Geometry: see drawing. Coordinates: mm, zero at the bounding-box minimum. A direction names the side the tool comes from. Round coordinates to 2 decimals unless told otherwise and drop trailing zeros. Loops run counter-clockwise (first coordinate to the right, second up) from the corner with the lowest first, then second, coordinate; pieces in that order, holes last. Notation, with made-up numbers: (31.25, 75.5) - (36.25, 75.5) arc R19 cw to (36.25, 96.5) - close; hole circle Ø2 at (65, 34). An arc over 180 degrees is marked (long way). Write item = value, one per line. Start each with the question number.
Item 1: Draft query along X for the marked faces 1, 2, 3 and 4. Return one class per face: pulls with the +X half, pulls with the -X half, needs draft (parallel to the pull), parting line crosses it, or undercut.
Item 2: Access query for the marked faces 5 and 6. Directions: +Z, -Z, +X, -X, +Y, -Y. A direction counts if a zero-diameter tool reaches every point of the face in a straight line with its end or side. Return the directions, or none.
Item 3: Line query: line 1 (X direction, y = 56, z = 5.5); line 2 (Y direction, x = 4.5, z = 33); line 3 (Y direction, x = 50, z = 22). Output: solid intervals per line, ascending. Write a range as from..to.
Item 4: First-contact query: pin 1 (2.5 mm diameter, centred on x = 11, z = 16.5, fed in from +Y); pin 2 (2 mm diameter, centred on x = 43.5, z = 35, fed in from -Y); pin 3 (2 mm diameter, centred on y = 14, z = 31.5, fed in from -X); pin 4 (10.5 mm diameter, centred on y = 41.5, z = 14.5, fed in from +X). Flat tips, straight axial feed; report the tip coordinate or a pass-through.
Item 5: Section C-C (x = 28). Return loops of the section in (y, z).
Item 6: Section A-A (z = 16.5). Count the separate pieces of the cut face and the enclosed holes in it, plus the area to 3 significant figures.
Item 7: Section D-D (y = 67). Return loops of the section in (x, z).
Item 8: Section B-B (y = 49). Return loops of the section in (x, z), plus the area to 3 significant figures.
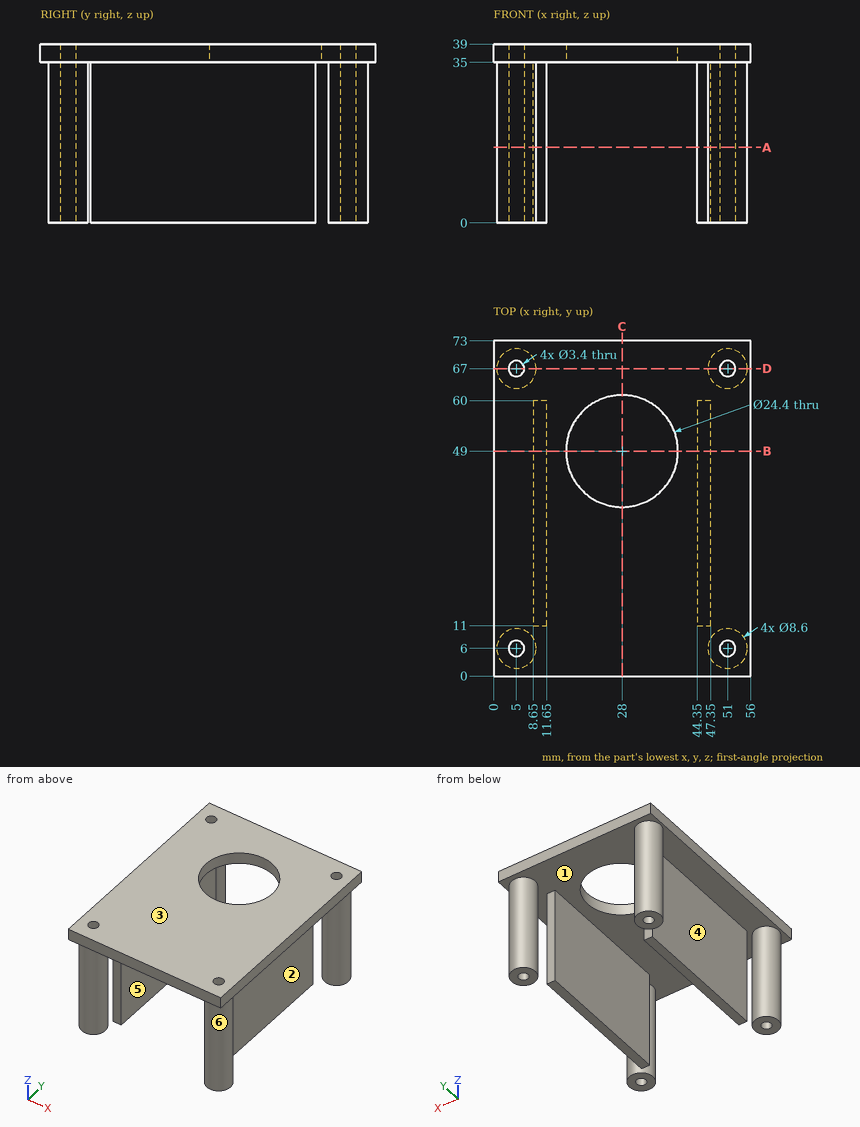
Taken from the geometry:
q1.face_1 = undercut
q1.face_2 = pulls with the +X half
q1.face_3 = needs draft
q1.face_4 = pulls with the -X half
q2.face_5 = -Z, +Y, -Y
q2.face_6 = -Z
q3.line_1 = 8.65..11.65, 44.35..47.35
q3.line_2 = 1.73..4.38, 7.62..10.27, 62.73..65.38, 68.62..71.27
q3.line_3 = 1.82..4.63, 7.37..10.18, 62.82..65.63, 68.37..71.18
q4.pin_1 = 60
q4.pin_2 = 0
q4.pin_3 = 8.65
q4.pin_4 = 47.35
q5.outline = (0, 35) - (36.8, 35) - (36.8, 39) - (0, 39) - close; (61.2, 35) - (73, 35) - (73, 39) - (61.2, 39) - close
q6.separate_pieces = 6
q6.enclosed_holes = 4
q6.area = 490 mm^2
q7.outline = (0, 35) - (0.7, 35) - (0.7, 0) - (3.3, 0) - (3.3, 39) - (0, 39) - close; (6.7, 0) - (9.3, 0) - (9.3, 35) - (46.7, 35) - (46.7, 0) - (49.3, 0) - (49.3, 39) - (6.7, 39) - close; (52.7, 0) - (55.3, 0) - (55.3, 35) - (56, 35) - (56, 39) - (52.7, 39) - close
q8.outline = (0, 35) - (8.65, 35) - (8.65, 0) - (11.65, 0) - (11.65, 35) - (15.8, 35) - (15.8, 39) - (0, 39) - close; (40.2, 35) - (44.35, 35) - (44.35, 0) - (47.35, 0) - (47.35, 35) - (56, 35) - (56, 39) - (40.2, 39) - close
q8.area = 336 mm^2
